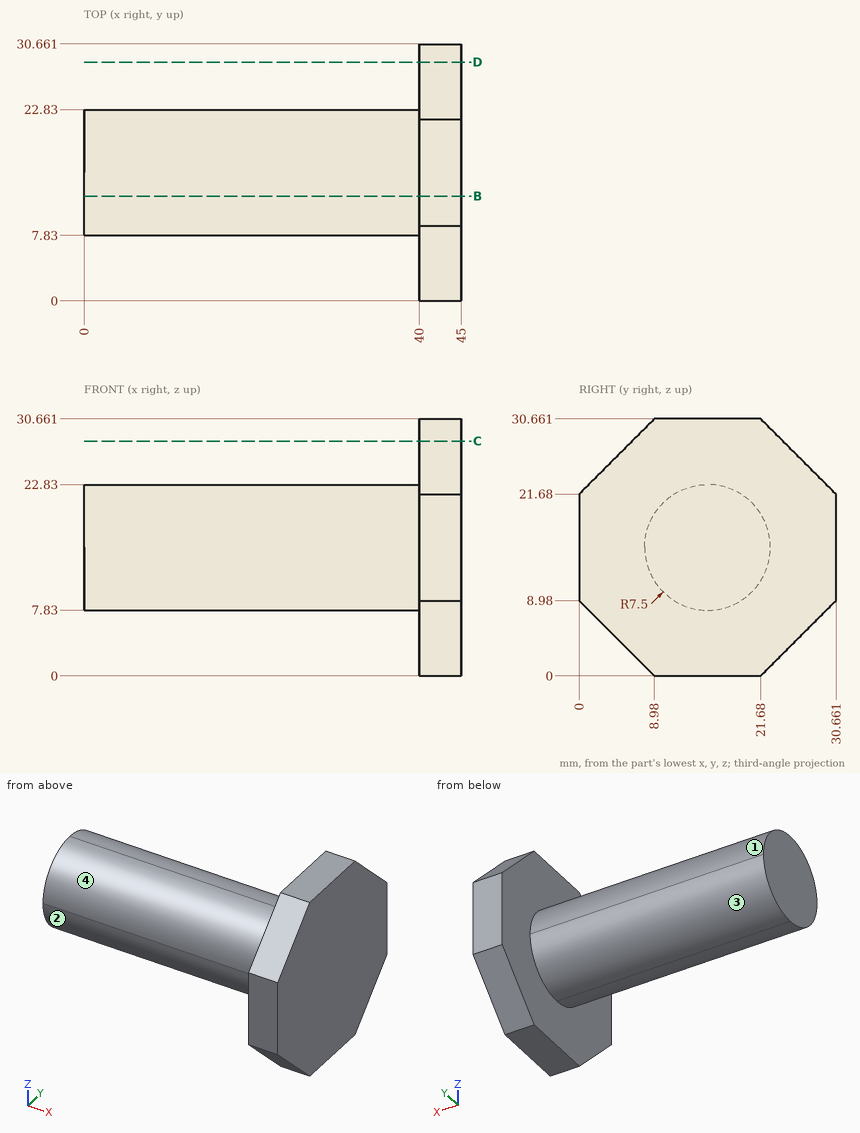
Source: three-view drawing plus pictorial views. Frame: mm from the lowest corner of the part. A direction names the side the tool comes from. Coordinates: 2 decimals unless noted, no trailing zeros. Loops run counter-clockwise (first coordinate to the right, second up) from the corner with the lowest first, then second, coordinate; pieces in that order, holes last. Notation, with made-up numbers: (-18.5, 8.25) -> (6.5, 8.25) arc R23 cw to (6.5, 16.25) -> close; hole circle Ø4 at (56.25, 45). An arc over 180 degrees is marked (long way). One line per item, written item: value.
(1) Cut plane C-C (z = 28). Output: boundary loops of the cut face in (x, y).
Answer below:
outline: (40, 6.32) -> (45, 6.32) -> (45, 24.34) -> (40, 24.34) -> close
(2) Ray query, line 1 along X through (y, z) = (23, 26.5); line 2 along Y through (x, z) = (31.5, 12); line 3 along Y through (x, z) = (8, 17). Return the intervals inside material, ascending.
Answer below:
line 1: x = 40 to 45
line 2: y = 8.61 to 22.05
line 3: y = 8.02 to 22.64
(3) Cut plane B-B (y = 12.5). Output: boundary loops of the cut face in (x, z) (1 decimal), then the cut area to 3 significant figures.
Answer below:
outline: (0, 8.4) -> (40, 8.4) -> (40, 0) -> (45, 0) -> (45, 30.7) -> (40, 30.7) -> (40, 22.3) -> (0, 22.3) -> close
area: 709 mm2
(4) Set-up query: the marked faces 1, 2, 3 and 4. Return all of +Z, -Z, +X, -X, +Y, -Y with unobstructed straight access to the full face (end or side cutting, diameter ignored); none if empty.
Answer below:
face 1: +Z, -X, +Y
face 2: -Z, -X, -Y
face 3: -Z, -X, +Y
face 4: +Z, -X, -Y
(5) Cut plane D-D (y = 28.5). Output: boundary loops of the cut face in (x, z).
Answer below:
outline: (40, 6.82) -> (45, 6.82) -> (45, 23.84) -> (40, 23.84) -> close
(6) Pin query (flat end, axial travel): pin 1 Ø10 at (x, y) = (13.5, 26) entering from +Z; pin 2 Ø1 at (x, y) = (13.5, 9) entering from -Z; pin 3 Ø1.5 at (x, y) = (39.5, 21.5) entering from +Z; pin 4 Ø10 at (x, z) = (21, 21.5) entering from -Y. Return the tip coordinate at first contact, or that it passes through.
Answer below:
pin 1: stops at z = 20.24
pin 2: stops at z = 10.61
pin 3: stops at z = 30.66
pin 4: stops at y = 7.92
